Part model, mm, in its own coordinate system. Coordinates: 2 decimals unless noted, no trailing zeros. Order: outer loops, then holes, each group sorted by start corner. A loop starts at its lowest first (then second) coordinate and runs counter-clockwise, first axis right, second up. Notation, with made-up numbers: (-0.75, -19.75) - (20.25, -19.75) arc R31 ccw to (20.25, 17.25) - close; hole circle Ø1 at (11.25, 79.5). An arc over 180 degrees is marked (long way). Use a Markdown table: item, result. Add a question column.
1) Saw through at A-A on y = 246. List the corners of the cut face in (x, z).
2) Saw through at B-B on z = 0.7. Count the separate pieces of the cut face and the enclosed holes in it, then the cut area to 3 significant figures.
3) Wall check: L1, parallel to X at y = 285, z = 0.95; L2, parallel to X at y = 170, z = 0.55; L3, parallel to X at y = 135, z = 0.95. Give the ranges that are in metal, low to high. Write a range as [from, to].
4) Drop flat-ended pins along their axis: P1, Ø4, axis at x = 60, y = 170, coming from the +Z side; P2, Ø0.8, axis at x = 9.5, z = 0.5, coming from the -Y side. Give the stop position or say it passes through.
```python
from build123d import *

# Parameters (mm, degrees)
ESQUISSE1_W                  = 180
ESQUISSE1_H                  = 340
BOSS_EXTRU_1_DEPTH           = 1.5
ESQUISSE2_R                  = 2.25
ENL_V_MAT_EXTRU_1_DEPTH      = 1
ENL_V_MAT_EXTRU_1_DEPTH_BACK = 2.5
ESQUISSE3_W                  = 22.5
ESQUISSE3_H                  = 30
ENL_V_MAT_EXTRU_2_DEPTH      = 1
ENL_V_MAT_EXTRU_2_DEPTH_BACK = 2.5
CONG_1_R                     = 10
CONG_2_R                     = 3
ESQUISSE4_W                  = 10
ESQUISSE4_H                  = 202
ENL_V_MAT_EXTRU_3_DEPTH      = 1
ENL_V_MAT_EXTRU_3_DEPTH_BACK = 2.5
CONG_3_R                     = 3
CHANFREIN1_SIZE              = 20
CHANFREIN2_SIZE              = 20
ESQUISSE5_R                  = 2.25
ENL_V_MAT_EXTRU_4_DEPTH      = 2.5
ESQUISSE6_R                  = 2.25
ENL_V_MAT_EXTRU_5_DEPTH      = 1
ENL_V_MAT_EXTRU_5_DEPTH_BACK = 2.5
CONG_4_R                     = 3.5


with BuildPart() as part:
    # Esquisse1 → Boss.-Extru.1 (new body)
    with BuildSketch(Plane.XY):
        with Locations((90, 170)):
            Rectangle(ESQUISSE1_W, ESQUISSE1_H)
    extrude(amount=BOSS_EXTRU_1_DEPTH)

    # Esquisse2 → Enlèv. mat.-Extru.1 (cut, two sides)
    with BuildSketch(Plane.XY.offset(1.5)) as enl_v_mat_extru_1_sk:
        with Locations((40, 13)):
            Circle(ESQUISSE2_R)
        with Locations((140, 13)):
            Circle(ESQUISSE2_R)
    extrude(amount=ENL_V_MAT_EXTRU_1_DEPTH, mode=Mode.SUBTRACT)
    extrude(enl_v_mat_extru_1_sk.sketch, amount=-ENL_V_MAT_EXTRU_1_DEPTH_BACK, mode=Mode.SUBTRACT)

    # Esquisse3 → Enlèv. mat.-Extru.2 (cut, two sides)
    with BuildSketch(Plane.XY.offset(1.5)) as enl_v_mat_extru_2_sk:
        with Locations((11.25, 15)):
            Rectangle(ESQUISSE3_W, ESQUISSE3_H)
        with Locations((168.75, 15)):
            Rectangle(ESQUISSE3_W, ESQUISSE3_H)
    extrude(amount=ENL_V_MAT_EXTRU_2_DEPTH, mode=Mode.SUBTRACT)
    extrude(enl_v_mat_extru_2_sk.sketch, amount=-ENL_V_MAT_EXTRU_2_DEPTH_BACK, mode=Mode.SUBTRACT)

    # Congé1
    cong_1_edges = [part.edges().sort_by_distance(p)[0] for p in [
        (22.5, 30, 0.75),
        (157.5, 30, 0.75),
    ]]
    fillet(cong_1_edges, radius=CONG_1_R)

    # Congé2
    cong_2_edges = [part.edges().sort_by_distance(p)[0] for p in [
        (0, 30, 0.75),
        (22.5, 0, 0.75),
        (180, 30, 0.75),
        (157.5, 0, 0.75),
    ]]
    fillet(cong_2_edges, radius=CONG_2_R)

    # Esquisse4 → Enlèv. mat.-Extru.3 (cut, two sides)
    with BuildSketch(Plane.XY.offset(1.5)) as enl_v_mat_extru_3_sk:
        with Locations((100, 191)):
            Rectangle(ESQUISSE4_W, ESQUISSE4_H)
    extrude(amount=ENL_V_MAT_EXTRU_3_DEPTH, mode=Mode.SUBTRACT)
    extrude(enl_v_mat_extru_3_sk.sketch, amount=-ENL_V_MAT_EXTRU_3_DEPTH_BACK, mode=Mode.SUBTRACT)

    # Congé3
    cong_3_edges = [part.edges().sort_by_distance(p)[0] for p in [
        (95, 90, 0.75),
        (95, 292, 0.75),
        (105, 292, 0.75),
        (105, 90, 0.75),
    ]]
    fillet(cong_3_edges, radius=CONG_3_R)

    # Chanfrein1
    chanfrein1_edges = [part.edges().sort_by_distance(p)[0] for p in [
        (180, 340, 0.75),
    ]]
    chamfer(chanfrein1_edges, length=CHANFREIN1_SIZE)

    # Chanfrein2
    chanfrein2_edges = [part.edges().sort_by_distance(p)[0] for p in [
        (0, 340, 0.75),
    ]]
    chamfer(chanfrein2_edges, length=CHANFREIN2_SIZE)

    # Esquisse5 → Enlèv. mat.-Extru.4 (cut, through all)
    with BuildSketch(Plane.XY.offset(1.5)):
        with Locations((120, 270)):
            Circle(ESQUISSE5_R)
    extrude(amount=-ENL_V_MAT_EXTRU_4_DEPTH, mode=Mode.SUBTRACT)

    # Esquisse6 → Enlèv. mat.-Extru.5 (cut, two sides)
    with BuildSketch(Plane.XY.offset(1.5)) as enl_v_mat_extru_5_sk:
        with Locations((6, 285)):
            Circle(ESQUISSE6_R)
        with Locations((6, 68)):
            Circle(ESQUISSE6_R)
        with Locations((174, 68)):
            Circle(ESQUISSE6_R)
        with Locations((174, 285)):
            Circle(ESQUISSE6_R)
        with Locations((20, 170)):
            Circle(ESQUISSE6_R)
        with Locations((60, 170)):
            Circle(ESQUISSE6_R)
        with Locations((149.5, 332.5)):
            Circle(ESQUISSE6_R)
        with Locations((170.630835149, 318.762563133)):
            Circle(ESQUISSE6_R)
        with Locations((9.369164851, 318.762563133)):
            Circle(ESQUISSE6_R)
        with Locations((30.5, 332.5)):
            Circle(ESQUISSE6_R)
    extrude(amount=ENL_V_MAT_EXTRU_5_DEPTH, mode=Mode.SUBTRACT)
    extrude(enl_v_mat_extru_5_sk.sketch, amount=-ENL_V_MAT_EXTRU_5_DEPTH_BACK, mode=Mode.SUBTRACT)

    # Congé4
    cong_4_edges = [part.edges().sort_by_distance(p)[0] for p in [
        (160, 340, 0.75),
        (180, 320, 0.75),
        (0, 320, 0.75),
        (20, 340, 0.75),
    ]]
    fillet(cong_4_edges, radius=CONG_4_R)


solid = part.part
```
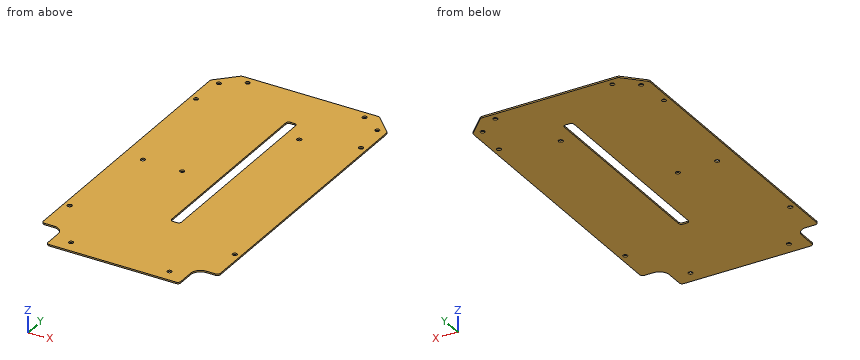
Results are:
| question | item | result |
|---|---|---|
| 1 | outline | (0, 0) - (95, 0) - (95, 1.5) - (0, 1.5) - close; (105, 0) - (180, 0) - (180, 1.5) - (105, 1.5) - close |
| 2 | separate pieces | 1 |
| 2 | enclosed holes | 14 |
| 2 | area | 57,300 mm2 |
| 3 | L1 | [0, 3.75], [8.25, 95], [105, 171.75], [176.25, 180] |
| 3 | L2 | [0, 17.75], [22.25, 57.75], [62.25, 95], [105, 180] |
| 3 | L3 | [0, 95], [105, 180] |
| 4 | P1 | through |
| 4 | P2 | y = 30 |
